```python
from build123d import *

# Parameters (mm, degrees)
BOSS_EXTRUDE1_DEPTH = 0.25
FILLET1_R           = 2
CUT_EXTRUDE1_REACH  = 2.5
SKETCH2_W           = 0.5
SKETCH2_H           = 2


with BuildPart() as part:
    # Sketch1 → Boss-Extrude1 (new body, symmetric)
    with BuildSketch(Plane(origin=(0, 0, 0), x_dir=(1, 0, 0), z_dir=(0, 1, 0))):
        with BuildLine():
            ThreePointArc((-8.5, 0), (-5.095377561, 5.095377561), (0, 8.5))
            ThreePointArc((0, 8.5), (5.095377561, 5.095377561), (8.5, 0))
            ThreePointArc((8.5, 0), (5.095377561, -5.095377561), (0, -8.5))
            ThreePointArc((0, -8.5), (-5.095377561, -5.095377561), (-8.5, 0))
        make_face()
    extrude(amount=BOSS_EXTRUDE1_DEPTH, both=True)

    # Fillet1
    fillet1_edges = [part.edges().sort_by_distance(p)[0] for p in [
        (-8.5, 0, 0),
        (0, 0, -8.5),
        (8.5, 0, 0),
        (0, 0, 8.5),
    ]]
    fillet(fillet1_edges, radius=FILLET1_R)

    # Sketch2 → Cut-Extrude1 (cut, up to next)
    with BuildSketch(Plane(origin=(0, 0.25, 0), x_dir=(1, 0, 0), z_dir=(0, 1, 0)), mode=Mode.PRIVATE) as cut_extrude1_sk1:
        with Locations((-6.25, 0)):
            Rectangle(SKETCH2_W, SKETCH2_H)
    cut_extrude1_tool1 = extrude(cut_extrude1_sk1.sketch, amount=-CUT_EXTRUDE1_REACH, mode=Mode.PRIVATE) & part.part
    add(cut_extrude1_tool1.solids().sort_by_distance((-6.25, 0.25, 0))[0], mode=Mode.SUBTRACT)
    # Sketch2 → Cut-Extrude1 (cut, up to next)
    with BuildSketch(Plane(origin=(0, 0.25, 0), x_dir=(1, 0, 0), z_dir=(0, 1, 0)), mode=Mode.PRIVATE) as cut_extrude1_sk2:
        with Locations((6.25, 0)):
            Rectangle(SKETCH2_W, SKETCH2_H)
    cut_extrude1_tool2 = extrude(cut_extrude1_sk2.sketch, amount=-CUT_EXTRUDE1_REACH, mode=Mode.PRIVATE) & part.part
    add(cut_extrude1_tool2.solids().sort_by_distance((6.25, 0.25, 0))[0], mode=Mode.SUBTRACT)


solid = part.part
```
Design review of the part built by this model. Coordinates are the model's own, in mm. Coordinates: 2 decimals unless noted, no trailing zeros. Order: outer loops, then holes, each group sorted by start corner. A loop starts at its lowest first (then second) coordinate and runs counter-clockwise, first axis right, second up.
1) Take a section at C-C, the plane x = -5.75. Give the boundary of the cut face in (y, z), and give its area (3 significant figures).
2) Take a section at B-B, the plane z = 2.25. Give the boundary of the cut face in (x, y).
3) Wall thickness on line 1 along X through (y, z) = (0, 0.75); line 2 along X through (y, z) = (-0.2, -6.25); line 3 along Z through (x, y) = (1.5, 0.1): over which ranges is each line inside the solid? List them lowest first.
4) Take a section at A-A, the plane y = -0.1. State how many separate pieces and enclosed holes the cut face has, and give its area (3 significant figures).
Returned:
1. outline: (-0.25, -4.4) - (0.25, -4.4) - (0.25, 4.4) - (-0.25, 4.4) - close
1. area: 4.40 mm2
2. outline: (-7.35, -0.25) - (7.35, -0.25) - (7.35, 0.25) - (-7.35, 0.25) - close
3. line 1: x = -8.16 to -6.5, -6 to 6, 6.5 to 8.16
3. line 2: x = -3.81 to 3.81
3. line 3: z = -7.78 to 7.78
4. separate pieces: 1
4. enclosed holes: 2
4. area: 181 mm2
